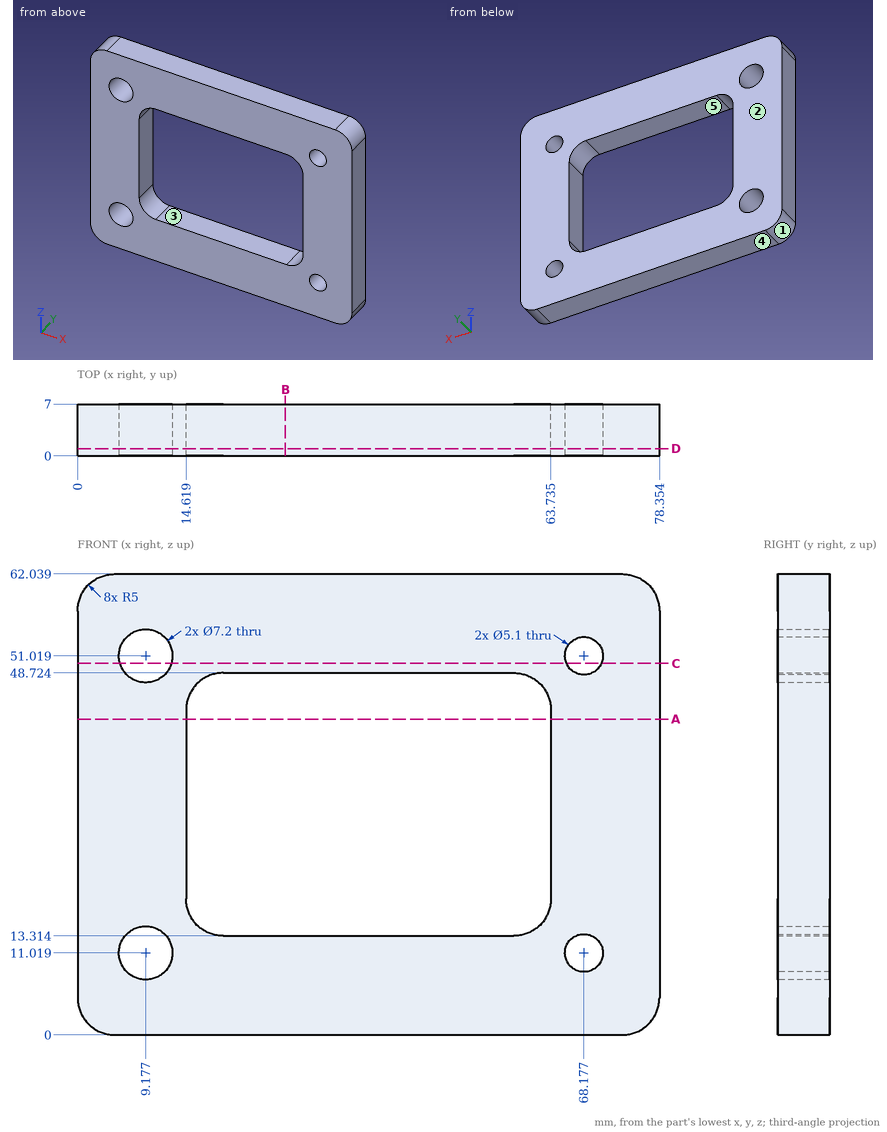
Print and shaded views of the part. All mm, measured from the part's lowest x, y and z. A direction names the side the tool comes from. Coordinates: 2 decimals unless noted, no trailing zeros. Loops run counter-clockwise (first coordinate to the right, second up) from the corner with the lowest first, then second, coordinate; pieces in that order, holes last. Notation, with made-up numbers: M 35.5,62.25 L 84.5,62.25 A5 ccw 84.5,67.25 Z; hole C 13.25,-9.5 d6. An arc over 180 degrees is marked long. Use a Markdown table: item, result. Add a question column.
Q1. Cut at C-C (z = 50). Write the cut outline in (x, y) (1 decimal).
Q2. Which spindle directions (+Z, -Z, +X, -X, +Y, -Y) get a long thin tool onto all of the face, cutting with end or side? Do the marked faces 4 and 5. Say none if no direction does.
Q3. Cut at B-B (x = 28). Write the cut outline in (y, z) (1 decimal).
Q4. Cut at A-A (z = 42.5). Write the cut outline in (x, y) (1 decimal).
Q5. Pin check, flat tip, straight feed: P1, Ø2, axis at y = 2, z = 30.5, coming from the -X side. Stop position of the tip, or through.
Q6. Cut at D-D (y = 1). Give the number of separate pieces and of enclosed holes in the cut face, and give its area (3 significant figures).
Q7. Mould opens along X. For the marked faces 1, 2 and 3 say: +X half, -X half, draft (parallel to the pull), parting line (faces both ways), or undercut.
Q8. Probe L1, parallel to X at y = 3.5, z = 51 (1 decimal); L2, parallel to X at y = 2.5, z = 42.5 (1 decimal); L3, parallel to Z at x = 27, y = 2.75 (1 decimal). List the from-to ranges inside material, lowest first.
Worked out:
| question | item | result |
|---|---|---|
| 1 | outline | M 0,0 L 5.7,0 L 5.7,7 L 0,7 Z; M 12.6,0 L 65.8,0 L 65.8,7 L 12.6,7 Z; M 70.5,0 L 78.4,0 L 78.4,7 L 70.5,7 Z |
| 2 | face 4 | -Z, +X, -X, +Y, -Y |
| 2 | face 5 | +Y, -Y |
| 3 | outline | M 0,0 L 7,0 L 7,13.3 L 0,13.3 Z; M 0,48.7 L 7,48.7 L 7,62 L 0,62 Z |
| 4 | outline | M 0,0 L 14.6,0 L 14.6,7 L 0,7 Z; M 63.7,0 L 78.4,0 L 78.4,7 L 63.7,7 Z |
| 5 | P1 | stops at x = 0 |
| 6 | separate pieces | 1 |
| 6 | enclosed holes | 5 |
| 6 | area | 3,000 mm2 |
| 7 | face 1 | -X half |
| 7 | face 2 | draft |
| 7 | face 3 | undercut |
| 8 | L1 | x = 0 to 5.6, 12.8 to 65.6, 70.7 to 78.4 |
| 8 | L2 | x = 0 to 14.6, 63.7 to 78.4 |
| 8 | L3 | z = 0 to 13.3, 48.7 to 62 |
